Can you work these out from the model? Positions are in its coordinate system, mm. A direction names the side the tool comes from. Round coordinates to 2 decimals unless told otherwise and drop trailing zeros. Order: outer loops, then holes, each group sorted by start corner. A loop starts at its lowest first (then second) coordinate and runs counter-clockwise, first axis right, second up. Notation, with made-up numbers: (-12.75, 52.5) -> (15.25, 52.5) arc R28 cw to (15.25, 78.5) -> close; hole circle Ø2 at (29.25, 89.25). An arc over 180 degrees is marked (long way). One line per item, written item: value.
Autodesk Inventor part; units mm, degrees
sketch "Sketch1" plane through (0, 0, 0) normal (0, 0, 1) x (1, 0, 0)
  line L0 (-250, 125) -> (250, 125)
  line L1 (250, 125) -> (250, -125)
  line L2 (250, -125) -> (-250, -125)
  line L3 (-250, -125) -> (-250, 125)
  line L4 (-250, 125) -> (250, -125) construction
  line L5 (250, 125) -> (-250, -125) construction
  point P0 (0, 0)
  point P1 (0, 0)
  dimension "d0" = 500
  dimension "d1" = 250
extrude "Extrusion1" add sketch "Sketch1" along normal mid plane 7
fillet "Fillet1" radius 2 4 edges at (250, 125, 0) (-250, 125, 0) (-250, -125, 0) (250, -125, 0)
sketch "Sketch2" plane through (0, 0, -3.5) normal (0, 0, -1) x (-1, 0, 0)
  line L0 (-102, -103) -> (-102, -57)
  line L1 (-102, -57) -> (-148, -57)
  line L2 (-148, -57) -> (-148, -103)
  line L3 (-148, -103) -> (-102, -103)
  line L4 (-105, -100) -> (-145, -100)
  line L5 (-145, -100) -> (-145, -60)
  line L6 (-145, -60) -> (-105, -60)
  line L7 (-105, -60) -> (-105, -100)
  line L8 (-101.5, -103.5) -> (-101.5, -56.5)
  line L9 (-101.5, -56.5) -> (-148.5, -56.5)
  line L10 (-148.5, -56.5) -> (-148.5, -103.5)
  line L11 (-148.5, -103.5) -> (-101.5, -103.5)
  line L12 (148, -103) -> (148, -57)
  line L13 (148, -57) -> (102, -57)
  line L14 (102, -57) -> (102, -103)
  line L15 (102, -103) -> (148, -103)
  line L16 (145, -100) -> (105, -100)
  line L17 (105, -100) -> (105, -60)
  line L18 (105, -60) -> (145, -60)
  line L19 (145, -60) -> (145, -100)
  line L20 (102, 103) -> (102, 57)
  line L21 (102, 57) -> (148, 57)
  line L22 (148, 57) -> (148, 103)
  line L23 (148, 103) -> (102, 103)
  line L24 (105, 100) -> (145, 100)
  line L25 (145, 100) -> (145, 60)
  line L26 (145, 60) -> (105, 60)
  line L27 (105, 60) -> (105, 100)
  line L28 (-148, 103) -> (-148, 57)
  line L29 (-148, 57) -> (-102, 57)
  line L30 (-102, 57) -> (-102, 103)
  line L31 (-102, 103) -> (-148, 103)
  line L32 (-145, 100) -> (-105, 100)
  line L33 (-105, 100) -> (-105, 60)
  line L34 (-105, 60) -> (-145, 60)
  line L35 (-145, 60) -> (-145, 100)
  line L36 (148.5, -103.5) -> (148.5, -56.5)
  line L37 (148.5, -56.5) -> (101.5, -56.5)
  line L38 (101.5, -56.5) -> (101.5, -103.5)
  line L39 (101.5, -103.5) -> (148.5, -103.5)
  line L40 (148.5, 56.5) -> (101.5, 56.5)
  line L41 (101.5, 56.5) -> (101.5, 103.5)
  line L42 (101.5, 103.5) -> (148.5, 103.5)
  line L43 (148.5, 103.5) -> (148.5, 56.5)
  line L44 (-101.5, 56.5) -> (-148.5, 56.5)
  line L45 (-148.5, 56.5) -> (-148.5, 103.5)
  line L46 (-148.5, 103.5) -> (-101.5, 103.5)
  line L47 (-101.5, 103.5) -> (-101.5, 56.5)
  point P0 (0, 0)
  dimension "d5" = 0.5
extrude "Extrusion2" cut sketch "Sketch2" against normal blind 3.5 contours L3 L2 L1 L0 | L4 L5 L6 L7 | L11 L10 L9 L8 | L15 L14 L13 L12 | L16 L17 L18 L19 | L23 L22 L21 L20 | L24 L25 L26 L27 | L31 L30 L29 L28 | L32 L33 L34 L35 | L39 L38 L37 L36 | L40 L41 L42 L43 | L44 L45 L46 L47
properties part number "sessao_07_04_002_001"
Q1. I want a section at C-C on y = 93. List the corners of the cut face in (x, z) for me.
Answers below:
outline: (-250, -3.5) -> (-148.5, -3.5) -> (-148.5, 0) -> (-101.5, 0) -> (-101.5, -3.5) -> (101.5, -3.5) -> (101.5, 0) -> (148.5, 0) -> (148.5, -3.5) -> (250, -3.5) -> (250, 3.5) -> (-250, 3.5) -> close
Q2. I want a section at A-A on z = -2. List the corners of the cut face in (x, y) for me, plus the area to 3 significant figures.
Answers below:
outline: (-250, -123) arc R2 ccw to (-248, -125) -> (248, -125) arc R2 ccw to (250, -123) -> (250, 123) arc R2 ccw to (248, 125) -> (-248, 125) arc R2 ccw to (-250, 123) -> close; hole (-148.5, -103.5) -> (-101.5, -103.5) -> (-101.5, -56.5) -> (-148.5, -56.5) -> close; hole (-148.5, 56.5) -> (-101.5, 56.5) -> (-101.5, 103.5) -> (-148.5, 103.5) -> close; hole (101.5, -103.5) -> (148.5, -103.5) -> (148.5, -56.5) -> (101.5, -56.5) -> close; hole (101.5, 56.5) -> (148.5, 56.5) -> (148.5, 103.5) -> (101.5, 103.5) -> close
area: 116,000 mm^2
Q3. We'd pull the mould along Y, two halves only. Please class faces 1 (the face through (-3, 2, 3.5)), 2 (the face through (-125, -80, 0)): released by +Y, released by -Y, zero draft, split by the parting line, or undercut.
Answers below:
face 1: zero draft
face 2: undercut
Q4. Will this pin go through, and if not, where does the flat tip stop? pin 1 Ø14 at (x, y) = (127.5, 82) entering from -Z.
Answers below:
pin 1: z = 0
Q5. On a 3-axis mill with a long thin cutter (end or side, diameter ignored), from which of +Z, -Z, +X, -X, +Y, -Y can I reach the whole of each face in a straight line? I mean faces 3 (the face through (-125, 80, 0)), 4 (the face through (-3, 2, -3.5)). Say none if no direction works.
Answers below:
face 3: -Z
face 4: -Z, +X, -X, +Y, -Y
Q6. I want a section at B-B on x = 113. List the corners of the cut face in (y, z) for me.
Answers below:
outline: (-125, -3.5) -> (-103.5, -3.5) -> (-103.5, 0) -> (-56.5, 0) -> (-56.5, -3.5) -> (56.5, -3.5) -> (56.5, 0) -> (103.5, 0) -> (103.5, -3.5) -> (125, -3.5) -> (125, 3.5) -> (-125, 3.5) -> close
Q7. Please list where these lines run through material, in increasing order: line 1 along Y through (x, z) = (-138, -2.5); line 2 along X through (y, z) = (66.5, -0.5); line 3 along Z through (x, y) = (-108, 70.5).
Answers below:
line 1: -125 to -103.5, -56.5 to 56.5, 103.5 to 125
line 2: -250 to -148.5, -101.5 to 101.5, 148.5 to 250
line 3: 0 to 3.5
